```python
from build123d import *

# Parameters (mm, degrees)
BOSS_EXTRUDE1_DEPTH = 4
CHAMFER1_SIZE       = 2
CHAMFER1_SIZE_2     = 1.414213562
CHAMFER2_SIZE       = 1


with BuildPart() as part:
    # Sketch1 → Boss-Extrude1 (new body)
    with BuildSketch(Plane.XY):
        Polygon((0, 4), (0, 0), (30.9, 0), (30.9, 4), (26.9, 4), (26.9, 8), (43, 8), (38.757359313, 12.242640687), (21.079689783, 29.920310217), (18.251262658, 27.091883092), (15.422835534, 29.920310217), (18.251262658, 32.748737342), (0, 51), (0, 36.857864376), (24.857864376, 12), (20.857864376, 12), (17.45, 12), (17.45, 8), (13.45, 8), (13.45, 12), (0, 12), (0, 8), (4, 8), (4, 4), align=None)
        Polygon((38.757359313, 12.242640687), (43, 8), (50.071067812, 15.071067812), (45.828427125, 19.313708499), align=None)
    extrude(amount=BOSS_EXTRUDE1_DEPTH)

    # Chamfer1
    # the kernel refuses this chamfer: 2, 1.414213562 mm, written as the material it adds along each edge
    with BuildSketch(Plane(origin=(38.757359313, 12.242640687, 0), x_dir=(-0.7262819568766827, 0.6873969152646646, 0), z_dir=(0, 0, 1))) as chamfer1_piece_1:
        Polygon((CHAMFER1_SIZE * 0.999621916911, -CHAMFER1_SIZE * 0.0274958766106), (-CHAMFER1_SIZE * 0.0274958766106, -CHAMFER1_SIZE * 0.999621916911), (0, 0), align=None)
    extrude(amount=4)
    # the kernel refuses this chamfer: 2, 1.414213562 mm, written as the material it takes off along each edge
    with BuildSketch(Plane(origin=(0, 51, -5.143365976), x_dir=(0.7262819568766843, -0.6873969152646628, 0), z_dir=(0, 0, 1))) as chamfer1_2_piece_1:
        Polygon((CHAMFER1_SIZE * 0.999621916911, -CHAMFER1_SIZE * 0.0274958766106), (CHAMFER1_SIZE_2 * 0.687396915446, -CHAMFER1_SIZE_2 * 0.726281957068), (0, 0), align=None)
    extrude(amount=14.286731952, mode=Mode.SUBTRACT)
    with BuildSketch(Plane(origin=(45.828427125, 19.313708499, -5.143365976), x_dir=(0.7262819568766831, -0.6873969152646641, 0), z_dir=(0, 0, 1)), Plane(origin=(50.071067812, 15.071067812, -5.143365976), x_dir=(-0.6873969152646642, -0.726281956876683, 0), z_dir=(0, 0, 1))) as chamfer1_2_piece_2:
        Polygon((CHAMFER1_SIZE * 0.999621916911, -CHAMFER1_SIZE * 0.0274958766106), (-CHAMFER1_SIZE * 0.0274958766106, -CHAMFER1_SIZE * 0.999621916911), (0, 0), align=None)
    extrude(amount=14.286731952, mode=Mode.SUBTRACT)
    with BuildSketch(Plane(origin=(0, 12, -5.143365976), x_dir=(-0.027495876610586365, -0.9996219169112968, 0), z_dir=(0, 0, 1))) as chamfer1_2_piece_3:
        Polygon((CHAMFER1_SIZE * 0.999621916911, CHAMFER1_SIZE * 0.0274958766106), (-CHAMFER1_SIZE * 0.0274958766106, CHAMFER1_SIZE * 0.999621916911), (0, 0), align=None)
    extrude(amount=14.286731952, mode=Mode.SUBTRACT)

    # Chamfer2
    chamfer2_edges = [part.edges().sort_by_distance(p)[0] for p in [
        (18.251262658, 32.748737342, 2),
        (21.079689783, 29.920310217, 2),
    ]]
    chamfer(chamfer2_edges, length=CHAMFER2_SIZE)


solid = part.part
```
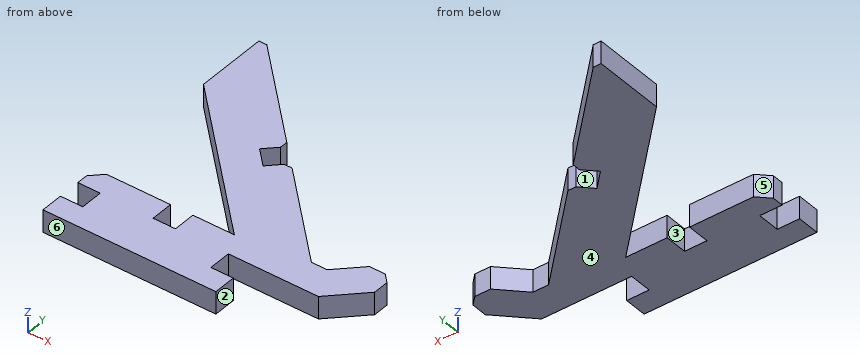
Read the model definition and answer for the solid it produces. Units are mm, in the model's axes. Face numbers are marked on the shaded views. A direction names the side the tool comes from. Give positions to 0.01 mm unless a question says otherwise; leave off trailing zeros. Order: outer loops, then holes, each group sorted by start corner. A loop starts at its lowest first (then second) coordinate and runs counter-clockwise, first axis right, second up. Notation, with made-up numbers: (-24, 30.25) -> (34, 30.25) arc R7 ccw to (34, 39.25) -> close; hole circle Ø4 at (-11, 8.5). An arc over 180 degrees is marked (long way). One line per item, written item: value. Start each with the question number.
(1) Straight lines are drawn through the part: L1, parallel to Y at x = 17.5, z = 0.45; L2, parallel to Y at x = 16.5, z = 3.15; L3, parallel to X at y = 14, z = 2.85. For each, find the intervals that lie inside material, in ascending order.
(2) Flat-ended cylindrical pins translate along their axes: P1, Ø0.7, axis at y = 33, z = 1, coming from the +X side; P2, Ø1.2, axis at x = 29.5, z = 1, coming from the +Y side; P3, Ø1.2, axis at x = 16, z = 1, coming from the +Y side. Find the tip coordinate at first contact, or state that the pin passes through.
(3) The part is cut by section A-A (x = 30). Determine the outline of the cut face in (y, z).
(4) A tool of negligible diameter and unlimited length cuts with its end or side. For the marked faces 1, 2 and 3, from which of +Z, -Z, +X, -X, +Y, -Y can it reach the whole face along a straight path? Write none if from no direction.
(5) For a pull along Y with two mould halves and no side action, classify the marked faces 4, 5 and 6 as released by +Y, released by -Y, zero draft, split by the parting line, or undercut.
(6) The part is cut by section C-C (y = 14.5). Determine the outline of the cut face in (x, z), and give its area (3 significant figures).
(7) The part is cut by section D-D (y = 44.5). Determine the outline of the cut face in (x, z), and give its area (3 significant figures).
Taken from the geometry:
1. L1: 0 to 12, 19.36 to 27.84, 32 to 33.5
1. L2: 0 to 8, 20.36 to 28.84, 31 to 34.5
1. L3: 22.86 to 37, 40.51 to 48.66
2. P1: x = 17.54
2. P2: y = 22.1
2. P3: y = 35.6
3. outline: (0, 0) -> (4, 0) -> (4, 4) -> (0, 4) -> close; (8, 0) -> (21, 0) -> (21, 4) -> (8, 4) -> close
4. face 1: +Z, -Z, +Y
4. face 2: +Z, -Z, +X, -Y
4. face 3: +Z, -Z
5. face 4: zero draft
5. face 5: undercut
5. face 6: released by -Y
6. outline: (22.36, 0) -> (36.5, 0) -> (36.5, 4) -> (22.36, 4) -> close; (41.01, 0) -> (48.66, 0) -> (48.66, 4) -> (41.01, 4) -> close
6. area: 87.1 mm^2
7. outline: (0, 0) -> (6.5, 0) -> (6.5, 4) -> (0, 4) -> close
7. area: 26.0 mm^2
